Could you check a few things on this drawing? It's one solid part, dimensions in mm from its lowest x, y, z. A direction names the side the tool comes from. Give positions to 0.01 mm unless a question says otherwise; leave off trailing zeros. Loops run counter-clockwise (first coordinate to the right, second up) from the corner with the lowest first, then second, coordinate; pieces in that order, holes last.
Q1. Suppose I cut it at C-C (y = 17.5). List the corners of the cut face in (x, z) for me, and give its area (3 significant figures).
Q2. For the marked faces 5, 6 and 7, which set-ups out of +Z, -Z, +X, -X, +Y, -Y let a thin tool reach every point of the face, with its end or its side?
Q3. I need wall thicknesses on probe 1 along Y at (x, z) = (3, 10); probe 2 along Z at (x, y) = (8.25, 4.5); probe 3 along Y at (x, z) = (11.75, 9.25). Which ranges of each line are inside material? Lowest first, please.
Q4. Suppose I cut it at B-B (x = 3). List the corners of the cut face in (y, z) for me.
Q5. Thinking about a two-plate mould opening in Y: for the marked faces 1, 2, 3 and 4, which applies, pulls with the +Y half, pulls with the -Y half, needs draft (parallel to the pull), parting line crosses it, or undercut?
Q6. Suppose I cut it at A-A (z = 10). List the corners of the cut face in (x, y) for me, and give its area (3 significant figures).
Q7. I'm going to push flat-ended pins straight in: P1, Ø6, axis at y = 18, z = 10, coming from the +X side; P2, Ø5, axis at x = 12.5, z = 7, coming from the +Y side. Where does each tip first touch, or does it pass through?
Q8. Suppose I cut it at D-D (x = 13). List the corners of the cut face in (y, z) for me, and give its area (3 significant figures).
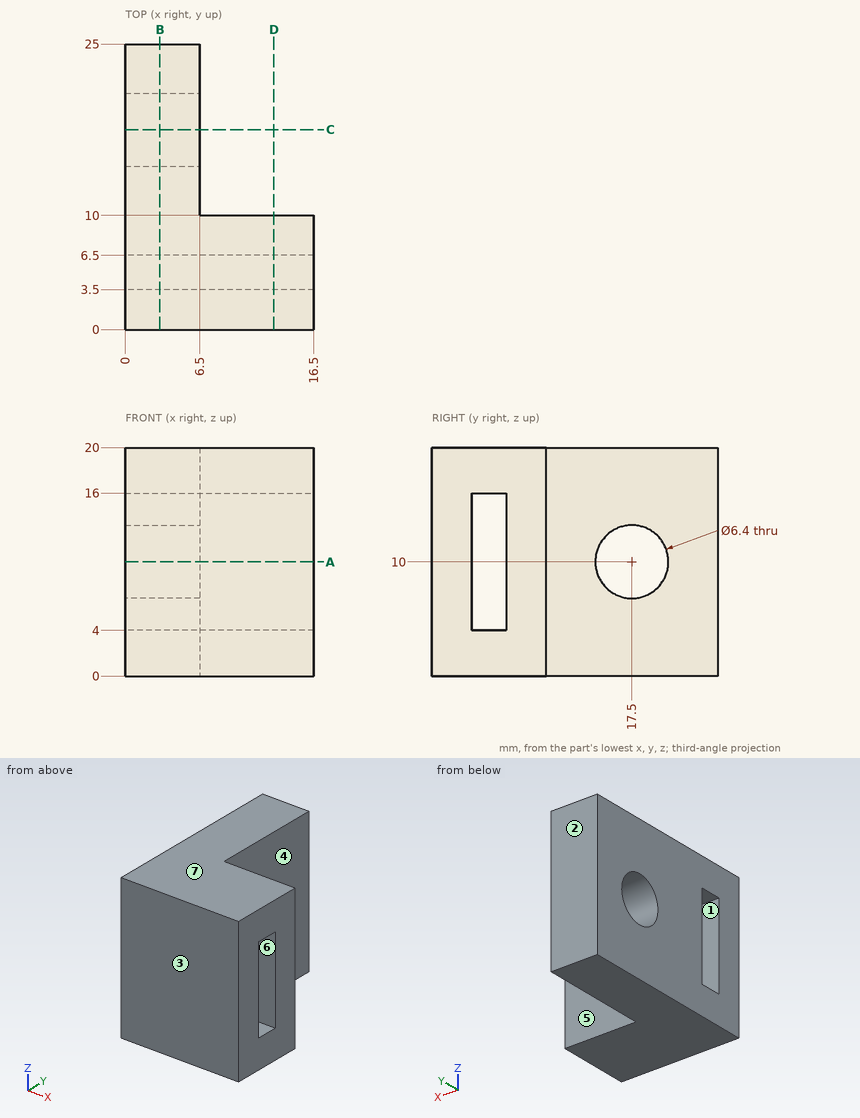
Solutions:
1. outline: (0, 0) - (6.5, 0) - (6.5, 6.8) - (0, 6.8) - close; (0, 13.2) - (6.5, 13.2) - (6.5, 20) - (0, 20) - close
1. area: 88.4 mm2
2. face 5: +Z, -Z, +X, +Y
2. face 6: +X, -X
2. face 7: +Z, +X, -X, +Y, -Y
3. probe 1: y = 0 to 3.5, 6.5 to 14.3, 20.7 to 25
3. probe 2: z = 0 to 4, 16 to 20
3. probe 3: y = 0 to 3.5, 6.5 to 10
4. outline: (0, 0) - (25, 0) - (25, 20) - (0, 20) - close; hole (3.5, 4) - (6.5, 4) - (6.5, 16) - (3.5, 16) - close; hole circle Ø6.4 at (17.5, 10)
5. face 1: undercut
5. face 2: pulls with the +Y half
5. face 3: pulls with the -Y half
5. face 4: needs draft
6. outline: (0, 0) - (16.5, 0) - (16.5, 3.5) - (0, 3.5) - close; (0, 6.5) - (16.5, 6.5) - (16.5, 10) - (6.5, 10) - (6.5, 14.3) - (0, 14.3) - close; (0, 20.7) - (6.5, 20.7) - (6.5, 25) - (0, 25) - close
6. area: 171 mm2
7. P1: stops at x = 6.5
7. P2: stops at y = 10
8. outline: (0, 0) - (10, 0) - (10, 20) - (0, 20) - close; hole (3.5, 4) - (6.5, 4) - (6.5, 16) - (3.5, 16) - close
8. area: 164 mm2
